Part print with two shaded views. Sizes in mm from the minimum x, y, z corner. A direction names the side the tool comes from. Round coordinates to 2 decimals unless told otherwise and drop trailing zeros. Write each loop counter-clockwise with the first axis right and the second up, starting at its lowest first coordinate (ties: lowest second). Pieces come first, ordered by that corner, then holes. Notation, with made-up numbers: (-18.75, 22) -> (1.25, 22) arc R15 ccw to (1.25, 35) -> close; hole circle Ø9 at (-32, 1). An arc over 180 degrees is marked (long way). Answer in a Markdown table with one row per item.
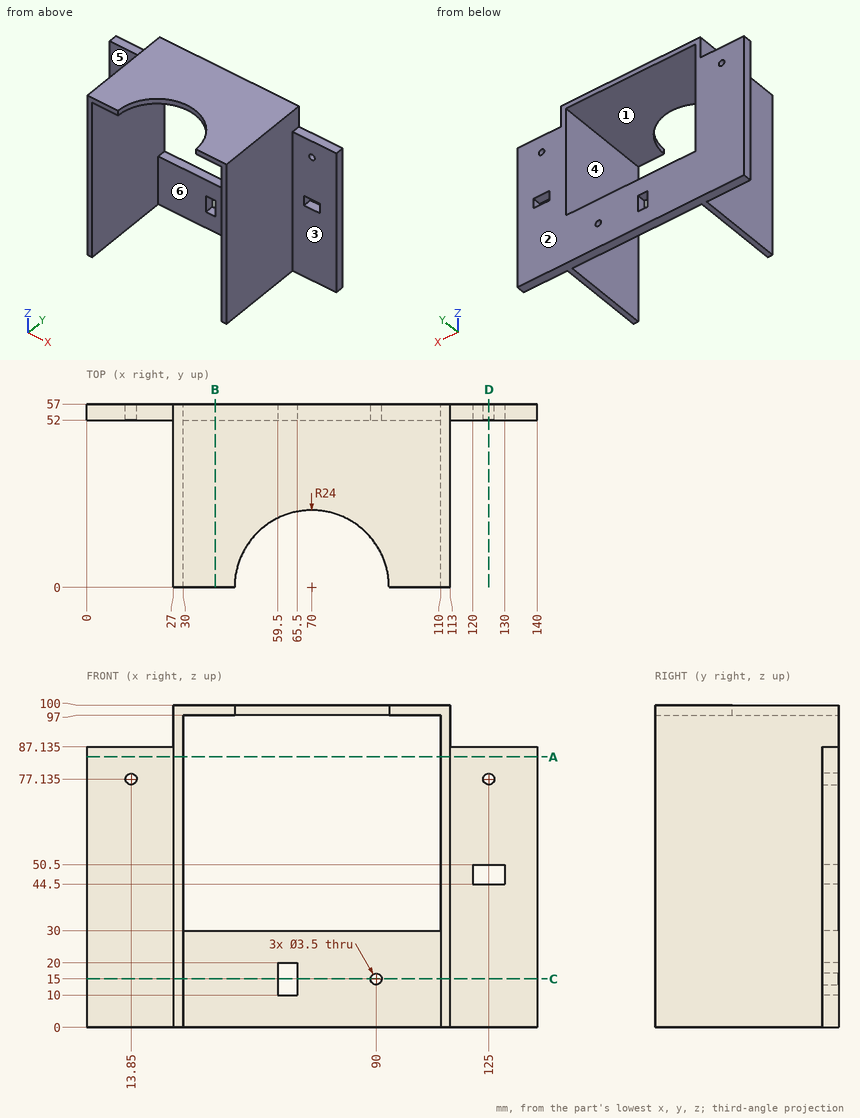
Q1. Saw through at D-D on x = 125. Write the cut outline in (y, z) (3 decimals), plus the area to 3 significant figures.
A:
| item | result |
|---|---|
| outline | (52, 0) -> (57, 0) -> (57, 44.5) -> (52, 44.5) -> close; (52, 50.5) -> (57, 50.5) -> (57, 75.385) -> (52, 75.385) -> close; (52, 78.885) -> (57, 78.885) -> (57, 87.135) -> (52, 87.135) -> close |
| area | 388 mm² |
Q2. Wall check: line 1 (X direction, y = 55, z = 15); line 2 (Z direction, x = 90, y = 55.2); line 3 (Z direction, x = 125, y = 54.45) (3 decimals). Give the ranges that are in metal, low to high. Write a range as [from, to].
A:
| item | result |
|---|---|
| line 1 | [0, 59.5], [65.5, 88.25], [91.75, 140] |
| line 2 | [0, 13.25], [16.75, 30], [97, 100] |
| line 3 | [0, 44.5], [50.5, 75.385], [78.885, 87.135] |
Q3. Saw through at A-A on z = 84. Write the cut outline in (x, y).
A:
| item | result |
|---|---|
| outline | (0, 52) -> (27, 52) -> (27, 0) -> (30, 0) -> (30, 57) -> (0, 57) -> close; (110, 0) -> (113, 0) -> (113, 52) -> (140, 52) -> (140, 57) -> (110, 57) -> close |
Q4. Saw through at B-B on x = 40. Write the cut outline in (y, z), plus the area to 3 significant figures.
A:
| item | result |
|---|---|
| outline | (0, 97) -> (57, 97) -> (57, 100) -> (0, 100) -> close; (52, 0) -> (57, 0) -> (57, 30) -> (52, 30) -> close |
| area | 321 mm² |
Q5. Drop flat-ended pins along their axis: P1, Ø12, axis at x = 48, y = 45, coming from the -Z side; P2, Ø1, axis at y = 48, z = 83.5, coming from the +X side; P3, Ø10, axis at x = 87.5, z = 22, coming from the -Y side; P4, Ø3, axis at x = 125, z = 77.13, coming from the -Y side. Give the stop position or say it passes through.
A:
| item | result |
|---|---|
| P1 | z = 97 |
| P2 | x = 113 |
| P3 | y = 52 |
| P4 | through |
Q6. Saw through at C-C on z = 15. Write the cut outline in (x, y).
A:
| item | result |
|---|---|
| outline | (0, 52) -> (27, 52) -> (27, 0) -> (30, 0) -> (30, 52) -> (59.5, 52) -> (59.5, 57) -> (0, 57) -> close; (65.5, 52) -> (88.25, 52) -> (88.25, 57) -> (65.5, 57) -> close; (91.75, 52) -> (110, 52) -> (110, 0) -> (113, 0) -> (113, 52) -> (140, 52) -> (140, 57) -> (91.75, 57) -> close |
Q7. Two-plate mould, pull along X, no slides. Class the marked faces 4, 5 and 6: released by +X, released by -X, zero draft, split by the parting line, or undercut.
A:
| item | result |
|---|---|
| face 4 | undercut |
| face 5 | zero draft |
| face 6 | undercut |
Q8. Which spindle directions (+Z, -Z, +X, -X, +Y, -Y) get a long thin tool onto all of the face, cutting with end or side? Do the marked faces 1, 2 and 3. Say none if no direction does.
A:
| item | result |
|---|---|
| face 1 | +Y, -Y |
| face 2 | +Z, -Z, +X, -X, +Y |
| face 3 | +Z, -Z, +X, -Y |
